Input: part model. Units: mm. Frame: model coordinates. Face numbers are marked on the shaded views. A direction names the side the tool comes from. Coordinates: 2 decimals unless noted, no trailing zeros. Write each loop counter-clockwise with the first axis right and the second up, starting at its lowest first coordinate (ties: lowest second). Pieces come first, ordered by that corner, then holes. Notation, with made-up numbers: (-9, 12.25) - (50, 12.25) arc R8 cw to (50, 16.25) - close; hole circle Ø10 at (34, 33). An arc over 180 degrees is marked (long way). Use CSV: the item, a comma, the result in double quotes.
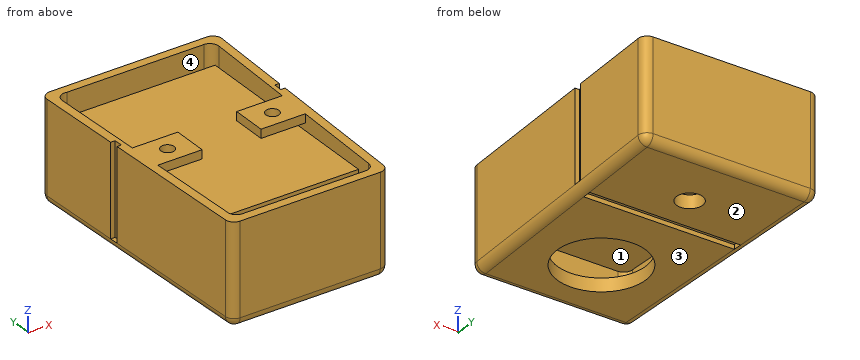
```python
from build123d import *

# Parameters (mm, degrees)
SKETCH1_R           = 3.75
SKETCH1_R_2         = 12.75
BOSS_EXTRUDE1_DEPTH = 3.81
BOSS_EXTRUDE3_DEPTH = 25.4
BOSS_EXTRUDE4_DEPTH = 2.54
FILLET1_R           = 2.54
BOSS_EXTRUDE6_DEPTH = 2.54
SKETCH9_R           = 1.905
CUT_EXTRUDE1_DEPTH  = 2.54
CUT_EXTRUDE2_DEPTH  = 1.27
SKETCH11_W          = 26.67
SKETCH11_H          = 2.54
CUT_EXTRUDE3_DEPTH  = 1.27
SKETCH12_W          = 26.67
SKETCH12_H          = 2.54
CUT_EXTRUDE4_DEPTH  = 1.27
SKETCH13_W          = 39.9796
SKETCH13_H          = 59.9948
BOSS_EXTRUDE7_DEPTH = 10.16


with BuildPart() as part:
    # Sketch1 → Boss-Extrude1 (new body)
    with BuildSketch(Plane.XY):
        with BuildLine():
            Line((-22.77090231, 76.154735329), (22.77090231, 76.154735329))
            ThreePointArc((22.77090231, 76.154735329), (24.597640016, 75.379566583), (25.309393487, 73.527199387))
            Line((25.309393487, 73.527199387), (22.858491178, 2.452464058))
            ThreePointArc((22.858491178, 2.452464058), (22.084831254, 0.713262294), (20.32, 0))
            Line((20.32, 0), (-20.32, 0))
            ThreePointArc((-20.32, 0), (-22.084831254, 0.713262294), (-22.858491178, 2.452464058))
            Line((-22.858491178, 2.452464058), (-25.309393487, 73.527199387))
            ThreePointArc((-25.309393487, 73.527199387), (-24.597640016, 75.379566583), (-22.77090231, 76.154735329))
        make_face()
        with Locations((0, 58.539610149)):
            Circle(SKETCH1_R, mode=Mode.SUBTRACT)
        with Locations((0, 21.622308918)):
            Circle(SKETCH1_R_2, mode=Mode.SUBTRACT)
    extrude(amount=BOSS_EXTRUDE1_DEPTH)

    # Sketch4 → Boss-Extrude3 (add)
    with BuildSketch(Plane.XY.offset(3.81)):
        with BuildLine():
            Line((-22.77090231, 76.154735329), (22.77090231, 76.154735329))
            ThreePointArc((22.77090231, 76.154735329), (24.597640016, 75.379566583), (25.309393487, 73.527199387))
            Line((25.309393487, 73.527199387), (22.858491178, 2.452464058))
            ThreePointArc((22.858491178, 2.452464058), (22.084831254, 0.713262294), (20.32, 0))
            Line((20.32, 0), (-20.32, 0))
            ThreePointArc((-20.32, 0), (-22.084831254, 0.713262294), (-22.858491178, 2.452464058))
            Line((-22.858491178, 2.452464058), (-25.309393487, 73.527199387))
            ThreePointArc((-25.309393487, 73.527199387), (-24.597640016, 75.379566583), (-22.77090231, 76.154735329))
        make_face()
        with BuildLine():
            Line((-19.541270744, 73.614735329), (20.141804619, 73.614735329))
            ThreePointArc((20.141804619, 73.614735329), (21.968542325, 72.839566583), (22.680295797, 70.987199387))
            Line((22.680295797, 70.987199387), (20.404569365, 4.992462187))
            ThreePointArc((20.404569365, 4.992462187), (19.630909441, 3.253260423), (17.866078187, 2.539998129))
            Line((17.866078187, 2.539998129), (-18.061159176, 2.539998129))
            ThreePointArc((-18.061159176, 2.539998129), (-19.78310781, 3.39559701), (-20.412160003, 5.212586245))
            Line((-20.412160003, 5.212586245), (-22.687990425, 71.210339105))
            ThreePointArc((-22.687990425, 71.210339105), (-21.690891162, 73.166710129), (-19.541270744, 73.614735329))
        make_face(mode=Mode.SUBTRACT)
    extrude(amount=BOSS_EXTRUDE3_DEPTH)

    # Sketch7 → Boss-Extrude4 (add)
    with BuildSketch(Plane.XY.offset(13.335)):
        with BuildLine():
            Line((-19.537731311, 73.614735329), (20.145344052, 73.614735329))
            ThreePointArc((20.145344052, 73.614735329), (21.972081758, 72.839566583), (22.68383523, 70.987199387))
            Line((22.68383523, 70.987199387), (20.408108798, 4.992462187))
            ThreePointArc((20.408108798, 4.992462187), (19.634448874, 3.253260423), (17.86961762, 2.539998129))
            Line((17.86961762, 2.539998129), (-18.057619743, 2.539998129))
            ThreePointArc((-18.057619743, 2.539998129), (-19.730779532, 3.364707915), (-20.389382819, 5.109944754))
            Line((-20.389382819, 5.109944754), (-22.665213241, 71.107697614))
            ThreePointArc((-22.665213241, 71.107697614), (-21.714144758, 73.125513756), (-19.537731311, 73.614735329))
        make_face()
    extrude(amount=BOSS_EXTRUDE4_DEPTH)

    # Fillet1
    fillet1_edges = [part.edges().sort_by_distance(p)[0] for p in [
        (-22.084831254, 0.713262294, 0),
        (-24.083942332, 37.989831723, 0),
        (-24.597640016, 75.379566583, 0),
        (0, 76.154735329, 0),
        (24.597640016, 75.379566583, 0),
        (24.083942332, 37.989831723, 0),
        (22.084831254, 0.713262294, 0),
        (0, 0, 0),
    ]]
    fillet(fillet1_edges, radius=FILLET1_R)

    # Sketch8 → Boss-Extrude6 (add)
    with BuildSketch(Plane.XY.offset(29.21)):
        Polygon((-21.717608556, 43.069831723), (-8.531459132, 43.069831723), (-8.531459132, 32.909831723), (-21.367256671, 32.909831723), align=None)
        Polygon((8.531459132, 32.909831723), (21.367256671, 32.909831723), (21.717608556, 43.069831723), (8.531459132, 43.069831723), align=None)
    extrude(amount=-BOSS_EXTRUDE6_DEPTH)

    # Sketch9 → Cut-Extrude1 (cut)
    with BuildSketch(Plane.XY.offset(29.21)):
        with Locations((-15.036945873, 37.989831723)):
            Circle(SKETCH9_R)
        with Locations((15.237744036, 37.820383377)):
            Circle(SKETCH9_R)
    extrude(amount=-CUT_EXTRUDE1_DEPTH, mode=Mode.SUBTRACT)

    # Sketch10 → Cut-Extrude2 (cut)
    with BuildSketch(Plane(origin=(0, 0, 0), x_dir=(-1, 0, 0), z_dir=(0, 0, -1))):
        Polygon((-21.897084176, 48.274519863), (21.897084176, 48.274519863), (21.809496204, 45.734519863), (-21.809496204, 45.734519863), align=None)
    extrude(amount=-CUT_EXTRUDE2_DEPTH, mode=Mode.SUBTRACT)

    # Sketch11 → Cut-Extrude3 (cut)
    with BuildSketch(Plane(origin=(-22.746873247, -0.784390739, 0), x_dir=(0, 0, 1), z_dir=(-0.999405975, -0.034462969, 0))):
        with Locations((15.875, 47.745550873)):
            Rectangle(SKETCH11_W, SKETCH11_H)
    extrude(amount=-CUT_EXTRUDE3_DEPTH, mode=Mode.SUBTRACT)

    # Sketch12 → Cut-Extrude4 (cut)
    with BuildSketch(Plane(origin=(22.746873247, -0.784390739, 0), x_dir=(0, 0, -1), z_dir=(0.999405975, -0.034462969, 0))):
        with Locations((-15.875, 47.745550873)):
            Rectangle(SKETCH12_W, SKETCH12_H)
    extrude(amount=-CUT_EXTRUDE4_DEPTH, mode=Mode.SUBTRACT)

    # Sketch13 → Boss-Extrude7 (add)
    with BuildSketch(Plane.XY.offset(15.875)):
        with Locations((-0.0762, 38.537335329)):
            Rectangle(SKETCH13_W, SKETCH13_H)
    extrude(amount=BOSS_EXTRUDE7_DEPTH)


solid = part.part
```
(1) Ray query, probe 1 along Y at (x, z) = (6, 24.5); probe 2 along Z at (x, y) = (-11, 38) (3 decimals); probe 3 along Z at (x, y) = (19, 25.5) (3 decimals). Return the intervals inside material, ascending. Write a range as from..to.
Check values:
probe 1,"0..2.54, 8.54..68.53, 73.61..76.15"
probe 2,"0..3.81, 13.335..26.035, 26.67..29.21"
probe 3,"0..3.81, 13.335..26.035"
(2) Reachability of the marked faces 1 and 2 from +Z, -Z, +X, -X, +Y, -Y: full face, straight path, thin tool, end or side. Return the list, or none.
Check values:
face 1,"none"
face 2,"-Z, +X, -X, +Y, -Y"
(3) Cut plane B-B on x = -14. State how many separate pieces and enclosed holes the cut face has, and give its area (3 significant figures).
Check values:
separate pieces,"3"
enclosed holes,"1"
area,"1,220 mm^2"
(4) Cut plane A-A on z = 19.5. Return loops of the section in (x, y), and give its area (3 significant figures).
Check values:
outline,"(-25.31, 73.53) - (-24.44, 48.2) - (-23.17, 48.25) - (-23.08, 45.71) - (-24.35, 45.66) - (-22.86, 2.45) arc R2.54 ccw to (-20.32, 0) - (20.32, 0) arc R2.54 ccw to (22.86, 2.45) - (24.35, 45.66) - (23.08, 45.71) - (23.17, 48.25) - (24.44, 48.2) - (25.31, 73.53) arc R2.54 ccw to (22.77, 76.15) - (-22.77, 76.15) arc R2.54 ccw to start; (-20.07, 8.54) - (19.91, 8.54) - (19.91, 68.53) - (-20.07, 68.53) - close; hole (-22.69, 71.21) - (-20.41, 5.21) arc R2.54 ccw to (-18.06, 2.54) - (17.87, 2.54) arc R2.54 ccw to (20.4, 4.99) - (22.68, 70.99) arc R2.54 ccw to (20.14, 73.61) - (-19.54, 73.61) arc R2.54 ccw to start"
area,"3,000 mm^2"
(5) Cut plane D-D on z = 8.75. Return loops of the section in (x, y).
Check values:
outline,"(-25.31, 73.53) - (-24.44, 48.2) - (-23.17, 48.25) - (-23.08, 45.71) - (-24.35, 45.66) - (-22.86, 2.45) arc R2.54 ccw to (-20.32, 0) - (20.32, 0) arc R2.54 ccw to (22.86, 2.45) - (24.35, 45.66) - (23.08, 45.71) - (23.17, 48.25) - (24.44, 48.2) - (25.31, 73.53) arc R2.54 ccw to (22.77, 76.15) - (-22.77, 76.15) arc R2.54 ccw to start; hole (-22.69, 71.21) - (-20.41, 5.21) arc R2.54 ccw to (-18.06, 2.54) - (17.87, 2.54) arc R2.54 ccw to (20.4, 4.99) - (22.68, 70.99) arc R2.54 ccw to (20.14, 73.61) - (-19.54, 73.61) arc R2.54 ccw to start"
(6) Pin query (flat end, axial travel): pin 1 Ø4 at (x, y) = (14.5, 43) entering from -Z; pin 2 Ø10 at (y, z) = (65, 15) entering from -X; pin 3 Ø2 at (x, y) = (11, 50.5) entering from +Z (3 decimals); pin 4 Ø5 at (y, z) = (24.5, 19.5) entering from -X (3 decimals). Return the tip coordinate at first contact, or that it passes through.
Check values:
pin 1,"z = 0"
pin 2,"x = -25.19"
pin 3,"z = 26.035"
pin 4,"x = -23.705"
(7) Draft query along X for the marked faces 3 and 4. Return one class per face: pulls with the +X half, pulls with the -X half, needs draft (parallel to the pull), parting line crosses it, or undercut.
Check values:
face 3,"needs draft"
face 4,"undercut"
